CAD build for the part. Positions are in the model's coordinates, mm. A direction names the side the tool comes from. Round coordinates to 2 decimals unless told otherwise and drop trailing zeros. Write each loop counter-clockwise with the first axis right and the second up, starting at its lowest first coordinate (ties: lowest second). Pieces come first, ordered by that corner, then holes. Notation, with made-up numbers: (64, 30) - (107, 30) arc R13 cw to (107, 45) - close; hole circle Ø8 at (-0.5, -34). An arc over 180 degrees is marked (long way). Use one line per item in the form item = value. Start each with the question number.
Item 1: Band-saw the part on D-D, the plane z = -41.5. List the corners of the cut face in (x, y).
Item 2: Band-saw the part on B-B, the plane z = 0. List the corners of the cut face in (x, y).
Item 3: Tool access for faces 1 (the flat face through (57.352, -1, 1)), 2 (the flat face through (-1, 0, -27)): list every direction of +Z, -Z, +X, -X, +Y, -Y with a clear straight run to the whole face (end or side of a thin tool).
Item 4: Band-saw the part on A-A, the plane x = 0. List the corners of the cut face in (y, z), and give its area (3 significant figures).
Item 5: Pull direction X, two halves, no side cores. Call faces 3 (the flat face through (-1, -1, 18.298)), 4 (the flat face through (-1, -3, -27)), 5 (the cylindrical face through (-13.77, -1.48, -61.99)), 6 (the flat face through (-1, -1, -16.702)): +X half, -X half, draft (parallel to the pull), parting line (faces both ways), or undercut.
Item 6: Pin check, flat tips, straight feed: pin 1 (0.9 mm diameter, centred on y = -1, z = 1, fed in from +X); pin 2 (0.9 mm diameter, centred on y = -2, z = -8, fed in from -X). Stop position of each tip, or through.
Item 7: Band-saw the part on C-C, the plane y = -1.65. List the corners of the cut face in (x, z).
Item 8: Drill centre lines: L1, parallel to X at y = -1.05, z = 5; L2, parallel to Z at x = -33.5, y = -2.6; L3, parallel to Z at x = 38, y = -2.8. Where is each one in solid material? Low to high.
from build123d import *

# Parameters (mm, degrees)
F0_R     = 63.5
F1_DEPTH = 3
F2_W     = 115
F2_H     = 35
F3_DEPTH = 3


with BuildPart() as f1:
    # F0 (on Front) → F1 (new body)
    with BuildSketch(Plane.XZ):
        Circle(F0_R)
    extrude(amount=F1_DEPTH)

    # F2 (on Front) → F3 (cut)
    with BuildSketch(Plane.XZ):
        with Locations((-0.148186, 0.797595)):
            Rectangle(F2_W, F2_H)
    extrude(amount=F3_DEPTH, mode=Mode.SUBTRACT)


solid = f1.part
Determined:
q1.outline = (-48.06, -3) - (48.06, -3) - (48.06, 0) - (-48.06, 0) - close
q2.outline = (-63.5, -3) - (-57.65, -3) - (-57.65, 0) - (-63.5, 0) - close; (57.35, -3) - (63.5, -3) - (63.5, 0) - (57.35, 0) - close
q3.face_1 = +Y, -Y
q3.face_2 = +Z, -Z, +X, -X, +Y
q4.outline = (-3, -63.5) - (0, -63.5) - (0, -16.7) - (-3, -16.7) - close; (-3, 18.3) - (0, 18.3) - (0, 63.5) - (-3, 63.5) - close
q4.area = 276 mm²
q5.face_3 = undercut
q5.face_4 = draft
q5.face_5 = parting line
q5.face_6 = undercut
q6.pin_1 = 63.5
q6.pin_2 = -63.05
q7.outline = circle Ø127 at (0, 0); hole (-57.65, -16.7) - (57.35, -16.7) - (57.35, 18.3) - (-57.65, 18.3) - close
q8.L1 = -63.3 to -57.65, 57.35 to 63.3
q8.L2 = -53.94 to -16.7, 18.3 to 53.94
q8.L3 = -50.87 to -16.7, 18.3 to 50.87
